The drawing under review shows one solid part. Ordinate dimensions are in mm from its lowest x, y, z. A direction names the side the tool comes from. Coordinates: 2 decimals unless noted, no trailing zeros. Order: outer loops, then holes, each group sorted by start corner. A loop starts at its lowest first (then second) coordinate and runs counter-clockwise, first axis right, second up.
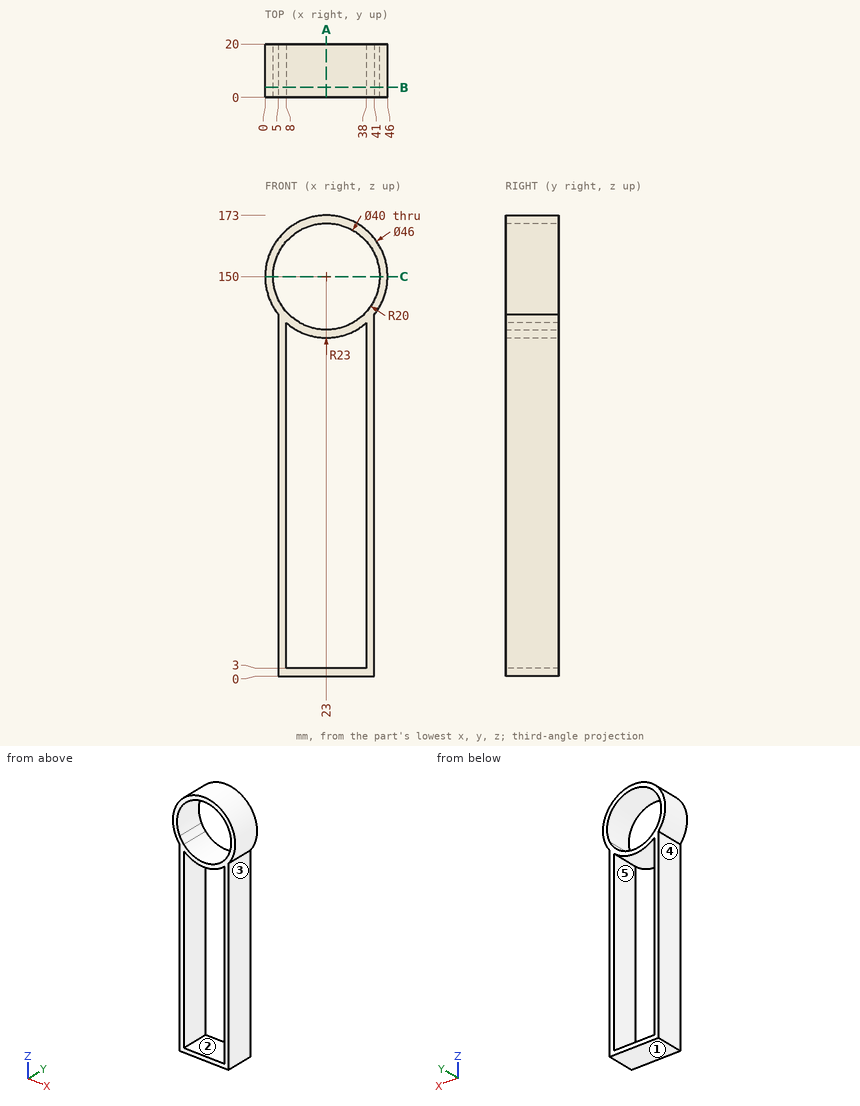
1. Clearance check with flat-ended pins moving along their axes: pin 1 Ø2 at (y, z) = (8.5, 85.5) entering from +X; pin 2 Ø3 at (y, z) = (17, 96) entering from -X; pin 3 Ø6 at (y, z) = (2.5, 142.5) entering from +X. State where each tip first meets the part, or that it passes through.
Answer below:
pin 1: stops at x = 41
pin 2: stops at x = 5
pin 3: stops at x = 45.56
2. Take a section at B-B, the plane y = 3.75. Give the boundary of the cut face in (x, z), plus the area to 3 significant figures.
Answer below:
outline: (5, 0) - (41, 0) - (41, 135.68) arc R23 ccw (long way) to (5, 135.68) - close; hole circle Ø40 at (23, 150); hole (8, 3) - (38, 3) - (38, 132.56) arc R23 cw to (8, 132.56) - close
area: 1,300 mm2
3. The part is to be moulded in two halves that separate along Z. For the marked faces 1, 2 and 3, say which applies: +Z half, -Z half, draft (parallel to the pull), parting line (faces both ways), or undercut.
Answer below:
face 1: -Z half
face 2: undercut
face 3: draft
4. To check wall thickness, follow L1, parallel to Z at x = 23, y = 14.75; L2, parallel to X at y = 13.75, z = 40; L3, parallel to X at y = 15, z = 150. State the ranges of each line that lie inside material, in increasing order.
Answer below:
L1: z = 0 to 3, 127 to 130, 170 to 173
L2: x = 5 to 8, 38 to 41
L3: x = 0 to 3, 43 to 46
5. Take a section at A-A, the plane x = 23. Give the boundary of the cut face in (y, z), plus the area to 3 significant figures.
Answer below:
outline: (0, 0) - (20, 0) - (20, 3) - (0, 3) - close; (0, 127) - (20, 127) - (20, 130) - (0, 130) - close; (0, 170) - (20, 170) - (20, 173) - (0, 173) - close
area: 180 mm2
6. Machinability: for the marked faces 4 and 5, which of the approach directions +Z, -Z, +X, -X, +Y, -Y give a long, thin tool a straight path to every point of the face, cutting with its end or side? Answer none if there is none.
Answer below:
face 4: -Z, -X, +Y, -Y
face 5: +Y, -Y
7. Take a section at C-C, the plane z = 150. Give the boundary of the cut face in (x, y).
Answer below:
outline: (0, 0) - (3, 0) - (3, 20) - (0, 20) - close; (43, 0) - (46, 0) - (46, 20) - (43, 20) - close
